```python
from build123d import *

# Parameters (mm, degrees)
F0_R      = 10
F1_DEPTH  = 50
F5_D      = 6.48
F5_DEPTH  = 12
F5_TIP    = 1.9467884056
F6_D      = 6.48
F6_DEPTH  = 12
F6_TIP    = 1.9467884056
F7_D      = 6.48
F7_DEPTH  = 12
F7_TIP    = 1.9467884056
F8_D      = 6.48
F8_DEPTH  = 12
F8_TIP    = 1.9467884056
F9_D      = 5.2
F9_DEPTH  = 23
F9_TIP    = 1.5622376095
F10_D     = 5.2
F10_DEPTH = 23
F10_TIP   = 1.5622376095
F11_D     = 5.2
F11_DEPTH = 23
F11_TIP   = 1.5622376095
F12_D     = 5.2
F12_DEPTH = 23
F12_TIP   = 1.5622376095


with BuildPart() as f1:
    # F0 (on Front) → F1 (new body)
    with BuildSketch(Plane.XZ):
        Polygon((15, -20.5), (27, -20.5), (27, -9.5), (26, -8.5), (26, 14.5), (15, 14.5), (9, 20.5), (-9, 20.5), (-15, 14.5), (-26, 14.5), (-26, -8.5), (-27, -9.5), (-27, -20.5), (-15, -20.5), (-14, -20), (14, -20), align=None)
        with Locations((0, 0.5)):
            Circle(F0_R, mode=Mode.SUBTRACT)
    extrude(amount=F1_DEPTH)

    # F5
    with Locations(Plane(origin=(0, 0, -20.5), x_dir=(1, 0, 0), z_dir=(0, 0, -1))):
        with Locations((20, 45)):
            Hole(F5_D / 2, depth=F5_DEPTH)
            with Locations((0, 0, -(F5_DEPTH + F5_TIP / 2))):  # 118° drill point
                Cone(0, F5_D / 2, F5_TIP, mode=Mode.SUBTRACT)

    # F6
    with Locations(Plane(origin=(0, 0, -20.5), x_dir=(1, 0, 0), z_dir=(0, 0, -1))):
        with Locations((-20, 45)):
            Hole(F6_D / 2, depth=F6_DEPTH)
            with Locations((0, 0, -(F6_DEPTH + F6_TIP / 2))):  # 118° drill point
                Cone(0, F6_D / 2, F6_TIP, mode=Mode.SUBTRACT)

    # F7
    with Locations(Plane(origin=(0, 0, -20.5), x_dir=(1, 0, 0), z_dir=(0, 0, -1))):
        with Locations((20, 5)):
            Hole(F7_D / 2, depth=F7_DEPTH)
            with Locations((0, 0, -(F7_DEPTH + F7_TIP / 2))):  # 118° drill point
                Cone(0, F7_D / 2, F7_TIP, mode=Mode.SUBTRACT)

    # F8
    with Locations(Plane(origin=(0, 0, -20.5), x_dir=(1, 0, 0), z_dir=(0, 0, -1))):
        with Locations((-20, 5)):
            Hole(F8_D / 2, depth=F8_DEPTH)
            with Locations((0, 0, -(F8_DEPTH + F8_TIP / 2))):  # 118° drill point
                Cone(0, F8_D / 2, F8_TIP, mode=Mode.SUBTRACT)

    # F9
    with Locations(Plane.XY.offset(14.5)):
        with Locations((20, -45)):
            Hole(F9_D / 2, depth=F9_DEPTH)
            with Locations((0, 0, -(F9_DEPTH + F9_TIP / 2))):  # 118° drill point
                Cone(0, F9_D / 2, F9_TIP, mode=Mode.SUBTRACT)

    # F10
    with Locations(Plane.XY.offset(14.5)):
        with Locations((-20, -45)):
            Hole(F10_D / 2, depth=F10_DEPTH)
            with Locations((0, 0, -(F10_DEPTH + F10_TIP / 2))):  # 118° drill point
                Cone(0, F10_D / 2, F10_TIP, mode=Mode.SUBTRACT)

    # F11
    with Locations(Plane.XY.offset(14.5)):
        with Locations((-20, -5)):
            Hole(F11_D / 2, depth=F11_DEPTH)
            with Locations((0, 0, -(F11_DEPTH + F11_TIP / 2))):  # 118° drill point
                Cone(0, F11_D / 2, F11_TIP, mode=Mode.SUBTRACT)

    # F12
    with Locations(Plane.XY.offset(14.5)):
        with Locations((20, -5)):
            Hole(F12_D / 2, depth=F12_DEPTH)
            with Locations((0, 0, -(F12_DEPTH + F12_TIP / 2))):  # 118° drill point
                Cone(0, F12_D / 2, F12_TIP, mode=Mode.SUBTRACT)


solid = f1.part
```
Here's how the part is built. I have some questions about the finished solid (model axes, mm). A direction names the side the tool comes from. Coordinates: 2 decimals unless noted, no trailing zeros. Order: outer loops, then holes, each group sorted by start corner. A loop starts at its lowest first (then second) coordinate and runs counter-clockwise, first axis right, second up. Notation, with made-up numbers: (-17.75, 87.5) - (-12.75, 87.5) arc R27 ccw to (-12.75, 126.5) - close; hole circle Ø4 at (60, -25). An arc over 180 degrees is marked (long way). One line per question, with ' | ' between items.
(1) Suppose I cut it at D-D on y = -26. List the corners of the cut face in (x, z) for me, and give its area (3 significant figures).
Report:
outline: (-27, -20.5) - (-15, -20.5) - (-14, -20) - (14, -20) - (15, -20.5) - (27, -20.5) - (27, -9.5) - (26, -8.5) - (26, 14.5) - (15, 14.5) - (9, 20.5) - (-9, 20.5) - (-15, 14.5) - (-26, 14.5) - (-26, -8.5) - (-27, -9.5) - close; hole circle Ø20 at (0, 0.5) | area: 1,660 mm2
(2) Suppose I cut it at C-C on x = -20. List the corners of the cut face in (y, z) for me.
Report:
outline: (-50, -20.5) - (-48.24, -20.5) - (-48.24, -8.5) - (-47.6, -8.12) - (-47.6, 14.5) - (-50, 14.5) - close; (-42.4, -8.12) - (-41.76, -8.5) - (-41.76, -20.5) - (-8.24, -20.5) - (-8.24, -8.5) - (-7.6, -8.12) - (-7.6, 14.5) - (-42.4, 14.5) - close; (-2.4, -8.12) - (-1.76, -8.5) - (-1.76, -20.5) - (0, -20.5) - (0, 14.5) - (-2.4, 14.5) - close
(3) Will these pins go through, and if not, where does the flat tip stop? pin 1 (8.5 mm diameter, centred on x = -20, y = -5, fed in from -Z); pin 2 (7 mm diameter, centred on x = 20, y = -5, fed in from +Z); pin 3 (1.5 mm diameter, centred on y = -33.5, z = 8.5, fed in from +X); pin 4 (4 mm diameter, centred on x = 20, y = -45, fed in from -Z).
Report:
pin 1: stops at z = -20.5 | pin 2: stops at z = 14.5 | pin 3: stops at x = 26 | pin 4: passes through
(4) If we mould it in two halves opening along Y, with no side actions, what happens to faces 1 (the flat face through (12, -24.6, 17.5)), 2 (the cylindrical face through (-22.48, -4.22, 3.03)), 3 (the flat face through (6, -50, -9)), 4 (the flat face through (6, 0, -9))? For each: pulls with the +Y half, pulls with the -Y half, needs draft (parallel to the pull), parting line crosses it, or undercut.
Report:
face 1: needs draft | face 2: undercut | face 3: pulls with the -Y half | face 4: pulls with the +Y half
(5) Suppose I cut it at A-A on y = -5. State how many separate pieces and enclosed holes the cut face has, and give its area (3 significant figures).
Report:
separate pieces: 3 | enclosed holes: 1 | area: 1,260 mm2
(6) Suppose I cut it at B-B on z = 0.5. List the corners of the cut face in (x, y) for me, and give its area (3 significant figures).
Report:
outline: (-26, -50) - (-10, -50) - (-10, 0) - (-26, 0) - close; (10, -50) - (26, -50) - (26, 0) - (10, 0) - close; hole circle Ø5.2 at (-20, -45); hole circle Ø5.2 at (-20, -5); hole circle Ø5.2 at (20, -45); hole circle Ø5.2 at (20, -5) | area: 1,520 mm2
(7) If I drill on L1, parallel to X at y = -45, z = -12; L2, parallel to Y at x = 20, z = 8.25; L3, parallel to Y at x = -20, z = -11.25, over which ranges is the centre line in solid material (lowest first)?
Report:
L1: x = -27 to -23.24, -16.76 to 16.76, 23.24 to 27 | L2: y = -50 to -47.6, -42.4 to -7.6, -2.4 to 0 | L3: y = -50 to -48.24, -41.76 to -8.24, -1.76 to 0
(8) For faces 5 (the cylindrical face through (-22.993, -3.759, -14.416)), 6 (the flat face through (-20, -25, 14.5)), 7 (the flat face through (21, -25, 14.5)), which set-ups out of +Z, -Z, +X, -X, +Y, -Y let a thin tool reach every point of the face, with its end or its side?
Report:
face 5: -Z | face 6: +Z, -X, +Y, -Y | face 7: +Z, +X, +Y, -Y
